Autodesk Inventor part; units mm, degrees
ref_plane "YZ Plane" through (0, 0, 0) normal (1, 0, 0) x (0, 1, 0)
ref_plane "XZ Plane" through (0, 0, 0) normal (0, 1, 0) x (-1, 0, 0)
ref_plane "XY Plane" through (0, 0, 0) normal (0, 0, 1) x (1, 0, 0)
sketch "Sketch1" plane through (0, 0, 0) normal (0, 0, 1) x (1, 0, 0)
  line L0 (-40.6, 0) -> (243.6, 0)
  line L1 (0, -40) -> (0, 240)
  line L2 (0, 0) -> (203, 0)
  line L3 (203, 0) -> (203, 200)
  line L4 (203, 200) -> (0, 200)
  line L5 (0, 200) -> (0, 0)
  dimension "d0" = 203
  dimension "d1" = 200
extrude "Extrusion1" add sketch "Sketch1" along normal blind 50
chamfer "Chamfer1" distance 50 angle 45 1 edges at (101.5, 0, 50)
sketch "Sketch4" plane through (0, 50, 50) normal (0, -0.7071, 0.7071) x (1, 0, 0)
  line L0 (32.6771, -55.3553) -> (116.9718, -55.3553)
  line L1 (116.9718, -55.3553) -> (116.9718, -15.3553)
  line L2 (116.9718, -15.3553) -> (32.6771, -15.3553)
  line L3 (32.6771, -15.3553) -> (32.6771, -55.3553)
extrude "Extrusion4" cut sketch "Sketch4" against normal blind 3
properties part number "hotbody"
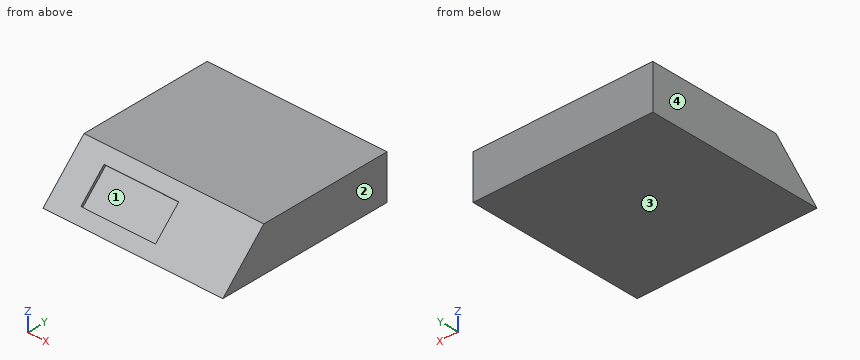
Geometry: final body of the model. Coordinates: model frame, mm. Face numbers are marked on the shaded views. Coordinates: 2 decimals unless noted, no trailing zeros. Order: outer loops, then holes, each group sorted by start corner. A loop starts at its lowest first (then second) coordinate and runs counter-clockwise, first axis right, second up.
Item 1: Section query B-B (z = 30). Output: boundary loops of the cut face in (x, y), then the cut area to 3 significant figures.
Answer:
outline: (0, 30) - (32.68, 30) - (32.68, 34.25) - (116.97, 34.25) - (116.97, 30) - (203, 30) - (203, 200) - (0, 200) - close
area: 34,200 mm2
Item 2: Material intervals for line 1 along Y through (x, z) = (44.5, 9); line 2 along Y through (x, z) = (172, 16.5); line 3 along Y through (x, z) = (12, 32.5), sorted ascending.
Answer:
line 1: y = 9 to 12.72, 13.25 to 200
line 2: y = 16.5 to 200
line 3: y = 32.5 to 200
Item 3: Draft query along X for the marked faces 1, 2, 3 and 4. Return one class per face: released by +X, released by -X, zero draft, split by the parting line, or undercut.
Answer:
face 1: undercut
face 2: released by +X
face 3: zero draft
face 4: released by -X
Item 4: Contact query for a flat-ended pin moving along its axis: P1, Ø6, axis at x = 72.5, y = 155, coming from the -Z side. Output: stop coordinate, or through.
Answer:
P1: stops at z = 0
